Autodesk Inventor part; units mm, degrees
ref_plane "YZ Plane" through (0, 0, 0) normal (1, 0, 0) x (0, 1, 0)
ref_plane "XZ Plane" through (0, 0, 0) normal (0, 1, 0) x (-1, 0, 0)
ref_plane "XY Plane" through (0, 0, 0) normal (0, 0, 1) x (1, 0, 0)
sketch "Sketch1" plane through (0, 0, 0) normal (0, 0, 1) x (1, 0, 0)
  line L0 (-14.5, -7) -> (17.5, -7)
  line L1 (17.5, -7) -> (17.5, 7)
  line L2 (17.5, 7) -> (-14.5, 7)
  line L3 (-14.5, 7) -> (-14.5, -7)
  line L4 (-14.5, -7) -> (17.5, 7) construction
  line L5 (17.5, -7) -> (-14.5, 7) construction
  line L6 (-14.5, 7) -> (-12.5, 7)
  line L7 (-12.5, 7) -> (-12.5, -7)
  line L8 (-12.5, -7) -> (-14.5, -7)
  line L9 (-14.5, -7) -> (-14.5, 7)
  line L10 (13.4907, 0) -> (-8.632, 0) construction
  line L11 (13.4907, 2) -> (-8.632, 2)
  line L12 (-8.632, -2) -> (13.4907, -2)
  arc A0 (13.4907, -2) -> (13.4907, 2) centre (13.4907, 0) ccw
  arc A1 (-8.632, 2) -> (-8.632, -2) centre (-8.632, 0) ccw
  point P0 (2.4294, 0)
  dimension "d0" = 32
  dimension "d1" = 14
  dimension "d4" = 2
  dimension "d6" = 4
extrude "Extrusion1" add sketch "Sketch1" along normal blind 2
extrude "Extrusion2" add sketch "Sketch1" along normal blind 25 contours L3 L2 L7 L0
fillet "Fillet1" radius 1 4 edges at (17.5, -7, 1) (17.5, 7, 1) (-13.5, 7, 25) (-13.5, -7, 25)
properties part number "actuator_backbone_fixings_for_measurements"
The listing builds one solid part. Answer for the finished solid, in the listing's coordinates (mm). A direction names the side the tool comes from. Give positions to 0.01 mm unless a question says otherwise; leave off trailing zeros. Write each loop counter-clockwise with the first axis right and the second up, starting at its lowest first coordinate (ties: lowest second). Pieces come first, ordered by that corner, then holes.
1) Section A-A (y = 0) is taken. Write down the section's boundary in (x, z).
2) A tool of negligible diameter and unlimited length cuts with its end or side. For faces 1 (the face through (15.49, 0.04, 0.99)), 2 (the face through (2, 3, 2)), 3 (the face through (1, 3, 0)), from which of +Z, -Z, +X, -X, +Y, -Y can it reach the whole face along a straight path? Write none if from no direction.
3) Section C-C (y = 3) is taken. Write down the section's boundary in (x, z), and give its area (3 significant figures).
4) Section D-D (z = 9) is taken. Write down the section's boundary in (x, y), and give its area (3 significant figures).
5) Find the intervals of material crossed by L1, parallel to X at y = -5, z = 14.5; L2, parallel to Z at x = -4, y = 5, in increasing order.
6) Given P1, Ø5, axis at x = 9, y = 4, coming from the +Z side; P2, Ø4, axis at x = -6.5, z = 4.5, coming from the +Y side, each flat-ended and moving along its own axis, determine where each tip first touches the part or whether it passes through.
7) Section B-B (x = 5.5) is taken. Write down the section's boundary in (y, z), and give its area (3 significant figures).
8) For a pull along X with two mould halves and no side action, classify faces 4 (the face through (-10.63, -0.04, 0.99)), 5 (the face through (3, 2, 1)), 6 (the face through (-13.486, -6.699, 24.715)), 7 (the face through (-12.5, 0, 13)) as pulls with the +X half, pulls with the -X half, needs draft (parallel to the pull), parting line crosses it, or undercut.
Response:
1. outline: (-14.5, 0) - (-10.63, 0) - (-10.63, 2) - (-12.5, 2) - (-12.5, 25) - (-14.5, 25) - close; (15.49, 0) - (17.5, 0) - (17.5, 2) - (15.49, 2) - close
2. face 1: +Z, -Z
2. face 2: +Z, +X, +Y, -Y
2. face 3: -Z, +X, -X, +Y, -Y
3. outline: (-14.5, 0) - (17.5, 0) - (17.5, 2) - (-12.5, 2) - (-12.5, 25) - (-14.5, 25) - close
3. area: 110 mm2
4. outline: (-14.5, -7) - (-12.5, -7) - (-12.5, 7) - (-14.5, 7) - close
4. area: 28.0 mm2
5. L1: x = -14.5 to -12.5
5. L2: z = 0 to 2
6. P1: stops at z = 2
6. P2: passes through
7. outline: (-7, 0) - (-2, 0) - (-2, 2) - (-7, 2) - close; (2, 0) - (7, 0) - (7, 2) - (2, 2) - close
7. area: 20.0 mm2
8. face 4: undercut
8. face 5: undercut
8. face 6: needs draft
8. face 7: pulls with the +X half
